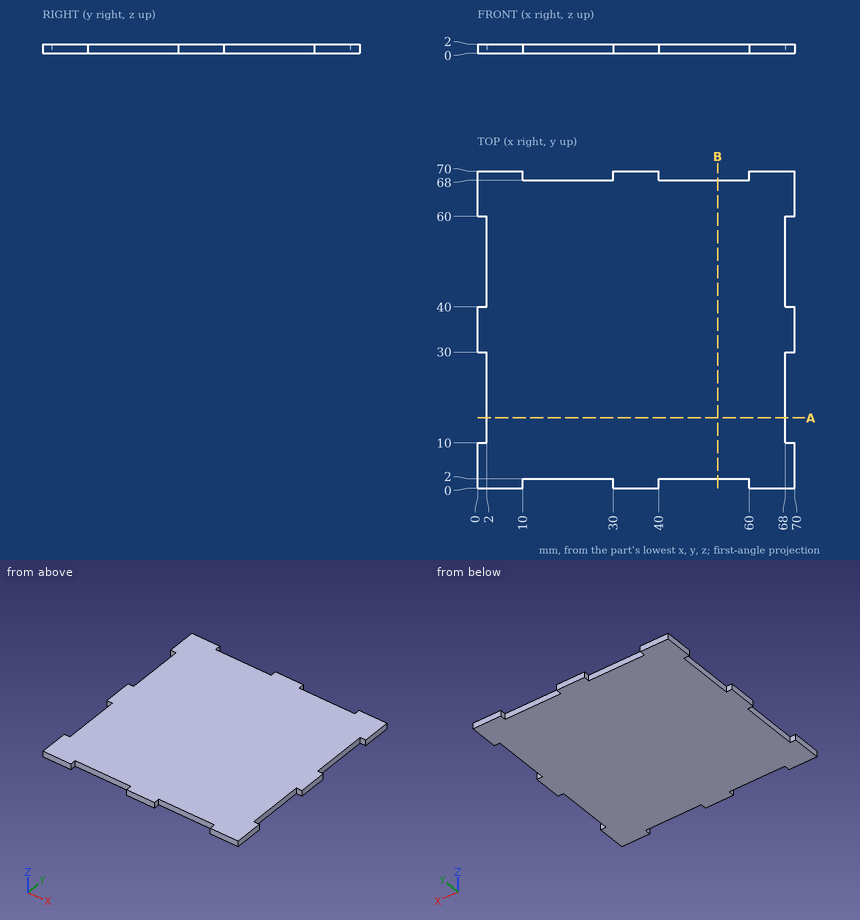
The figure shows three views and two pictorial views of one solid part (mm, origin at its lowest corner). Answer the questions. Coordinates: 2 decimals unless noted, no trailing zeros. Loops run counter-clockwise (first coordinate to the right, second up) from the corner with the lowest first, then second, coordinate; pieces in that order, holes last. Notation, with made-up numbers: (-10.75, 83.5) -> (22.25, 83.5) arc R26 cw to (22.25, 106.5) -> close; hole circle Ø6 at (28, 3.25). An arc over 180 degrees is marked (long way). Return JSON: item names as keys, results as strings. Group by question number.
(1) A cutting plane is placed at A-A on y = 15.5. Write down the section's boundary in (x, z).
(2) Find the intervals of material crossed by probe 1 along X at (y, z) = (42.5, 1), in increasing order. Write a range as from..to.
(3) Given pin 1 Ø0.6 at (y, z) = (47.5, 1.5) entering from -X; pin 2 Ø0.6 at (x, z) = (48, 1.5) entering from +Y; pin 3 Ø1 at (x, z) = (52, 1) entering from -Y, each flat-ended and moving along its own axis, determine where each tip first touches the part or whether it passes through.
The answers:
{
 "1": {"outline": "(2, 0) -> (68, 0) -> (68, 2) -> (2, 2) -> close"},
 "2": {"probe 1": "x = 2..68"},
 "3": {"pin 1": "stops at x = 2", "pin 2": "stops at y = 68", "pin 3": "stops at y = 2"}
}
